Verification items for the finished model (mm, model axes). Face numbers are marked on the shaded views. A direction names the side the tool comes from. Coordinates: 2 decimals unless noted, no trailing zeros. Loops run counter-clockwise (first coordinate to the right, second up) from the corner with the lowest first, then second, coordinate; pieces in that order, holes last. Notation, with made-up numbers: (9, -26.5) - (44, -26.5) arc R19 ccw to (44, -7.5) - close; hole circle Ø2 at (-26.5, 29.5). An arc over 180 degrees is marked (long way). One line per item, written item: value. Start each with the question number.
(1) Section check A-A (z = 10). Record the boundary of the cut face in (x, y), plus the area to 3 significant figures.
(2) Set-up check for the marked faces 1 and 2: record each of +Z, -Z, +X, -X, +Y, -Y from which the full face is reachable in a straight line by a thin tool's end or side.
(3) Thickness scan on probe 1 along X at (y, z) = (-19.5, -14); probe 2 along Y at (x, z) = (-6.5, 2.5); probe 3 along Z at (x, y) = (-7.5, -0.5). Record the ranges inside material, lowest first. Write a range as [from, to].
(4) Section check B-B (x = -11). Record the boundary of the cut face in (y, z), plus the area to 3 significant figures.
(5) Section check C-C (y = 0). Record the boundary of the cut face in (x, z).
(6) Section check D-D (x = 10.5). Record the boundary of the cut face in (y, z).
(7) Gauge pin test, flat ends, axial feed: P1, Ø12, axis at y = -21.5, z = 16, coming from the +X side; P2, Ø5, axis at x = 15.5, y = -4.5, coming from the -Z side; P3, Ø1, axis at x = -4.5, z = -12, coming from the -Y side. Record the tip position at first contact, or that the pin passes through.
```python
from build123d import *

# Parameters (mm, degrees)
F1_DEPTH = 20
F2_R     = 15
F3_DEPTH = 50


with BuildPart() as f1:
    # F0 (on Right) → F1 (new body)
    with BuildSketch(Plane.YZ):
        Polygon((-15.648834, -25.261711), (14.052867, -26.183143), (29.701701, -0.921432), (15.648834, 25.261711), (-14.052867, 26.183143), (-29.701701, 0.921432), align=None)
    extrude(amount=-F1_DEPTH)

    # F2 (on face) → F3 (join)
    with BuildSketch(Plane.YZ):
        Circle(F2_R)
    extrude(amount=F3_DEPTH)


solid = f1.part
```
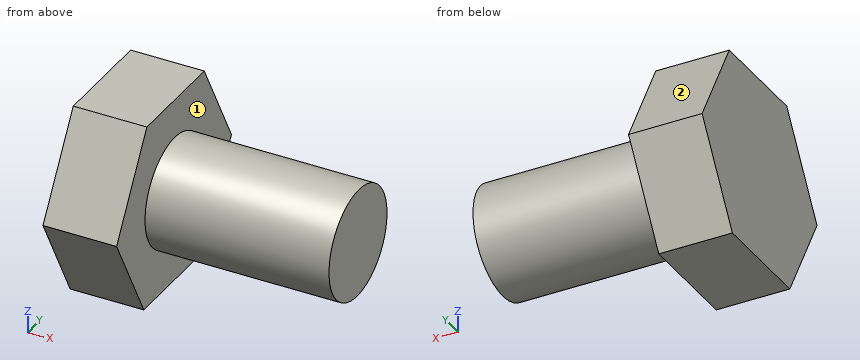
Responses:
1. outline: (-20, -24.08) - (0, -24.08) - (0, -11.18) - (50, -11.18) - (50, 11.18) - (0, 11.18) - (0, 23.84) - (-20, 23.84) - close
1. area: 2,080 mm²
2. face 1: +X
2. face 2: +Z, +X, -X, +Y
3. probe 1: x = [-20, 0]
3. probe 2: y = [-28.72, 27.87]
3. probe 3: z = [-25.73, 25.76]
4. outline: (-29.7, 0.92) - (-15.65, -25.26) - (14.05, -26.18) - (29.7, -0.92) - (15.65, 25.26) - (-14.05, 26.18) - close
4. area: 2,290 mm²
5. outline: (-20, -25.75) - (0, -25.75) - (0, -15) - (50, -15) - (50, 15) - (0, 15) - (0, 25.75) - (-20, 25.75) - close
6. outline: circle Ø30 at (0, 0)
7. P1: stops at x = 0
7. P2: stops at z = -14.87
7. P3: stops at y = -23.03
